from build123d import *

# Parameters (mm, degrees)
SKETCH1_R           = 12.25
BOSS_EXTRUDE1_DEPTH = 2.9
CUT_EXTRUDE1_REACH  = 364.631
SKETCH2_R           = 5
CUT_EXTRUDE2_REACH  = 364.631
SKETCH5_R           = 1.65
SKETCH6_R           = 9.75
SKETCH6_R_2         = 5
BOSS_EXTRUDE2_DEPTH = 3.72
SKETCH7_R           = 1.65
CUT_EXTRUDE3_DEPTH  = 3.72
SKETCH8_R           = 2.7
CUT_EXTRUDE4_DEPTH  = 2.5


with BuildPart() as part:
    # Sketch1 → Boss-Extrude1 (new body)
    with BuildSketch(Plane.XY):
        with Locations(Location((350.15, -0.367507575, 0), (0, 0, 180))):
            Circle(SKETCH1_R)
    extrude(amount=BOSS_EXTRUDE1_DEPTH)

    # Sketch2 → Cut-Extrude1 (cut, up to next)
    with BuildSketch(Plane.XY.offset(2.9), mode=Mode.PRIVATE) as cut_extrude1_sk1:
        with Locations((350.15, -0.367507575)):
            Circle(SKETCH2_R)
    cut_extrude1_tool1 = extrude(cut_extrude1_sk1.sketch, amount=-CUT_EXTRUDE1_REACH, mode=Mode.PRIVATE) & part.part
    add(cut_extrude1_tool1.solids().sort_by_distance((350.15, -0.367508, 2.9))[0], mode=Mode.SUBTRACT)

    # Sketch5 → Cut-Extrude2 (cut, up to next)
    with BuildSketch(Plane.XY.offset(2.9), mode=Mode.PRIVATE) as cut_extrude2_sk1:
        with Locations((343.05020627, -2.784722708)):
            Circle(SKETCH5_R)
    cut_extrude2_tool1 = extrude(cut_extrude2_sk1.sketch, amount=-CUT_EXTRUDE2_REACH, mode=Mode.PRIVATE) & part.part
    # Sketch5 → Cut-Extrude2 (cut, up to next)
    with BuildSketch(Plane.XY.offset(2.9), mode=Mode.PRIVATE) as cut_extrude2_sk2:
        with Locations((355.793266576, -5.30750174)):
            Circle(SKETCH5_R)
    cut_extrude2_tool2 = extrude(cut_extrude2_sk2.sketch, amount=-CUT_EXTRUDE2_REACH, mode=Mode.PRIVATE) & part.part
    # Sketch5 → Cut-Extrude2 (cut, up to next)
    with BuildSketch(Plane.XY.offset(2.9), mode=Mode.PRIVATE) as cut_extrude2_sk3:
        with Locations((351.606527153, 6.989701723)):
            Circle(SKETCH5_R)
    cut_extrude2_tool3 = extrude(cut_extrude2_sk3.sketch, amount=-CUT_EXTRUDE2_REACH, mode=Mode.PRIVATE) & part.part
    add(cut_extrude2_tool1.solids().sort_by_distance((343.050206, -2.784723, 2.9))[0], mode=Mode.SUBTRACT)
    add(cut_extrude2_tool2.solids().sort_by_distance((355.793267, -5.307502, 2.9))[0], mode=Mode.SUBTRACT)
    add(cut_extrude2_tool3.solids().sort_by_distance((351.606527, 6.989702, 2.9))[0], mode=Mode.SUBTRACT)

    # Sketch6 → Boss-Extrude2 (add)
    with BuildSketch(Plane(origin=(0, 0, 0), x_dir=(-1, 0, 0), z_dir=(0, 0, -1))):
        with Locations(Location((-350.15, -0.367507575, 0), (0, 0, 180))):
            Circle(SKETCH6_R)
        with Locations(Location((-350.15, -0.367507575, 0), (0, 0, 180))):
            Circle(SKETCH6_R_2, mode=Mode.SUBTRACT)
    extrude(amount=BOSS_EXTRUDE2_DEPTH)

    # Sketch7 → Cut-Extrude3 (cut)
    with BuildSketch(Plane.XY):
        with Locations((351.606527153, 6.989701723)):
            Circle(SKETCH7_R)
        with Locations((343.05020627, -2.784722708)):
            Circle(SKETCH7_R)
        with Locations((355.793266576, -5.30750174)):
            Circle(SKETCH7_R)
    extrude(amount=-CUT_EXTRUDE3_DEPTH, mode=Mode.SUBTRACT)

    # Sketch8 → Cut-Extrude4 (cut)
    with BuildSketch(Plane.XY.offset(2.9)):
        with Locations((351.606527153, 6.989701723)):
            Circle(SKETCH8_R)
        with Locations((355.793266576, -5.30750174)):
            Circle(SKETCH8_R)
        with Locations((343.05020627, -2.784722708)):
            Circle(SKETCH8_R)
    extrude(amount=-CUT_EXTRUDE4_DEPTH, mode=Mode.SUBTRACT)


solid = part.part
CAD build for the part. Positions are in the model's coordinates, mm. A direction names the side the tool comes from. Round coordinates to 2 decimals unless told otherwise and drop trailing zeros. Loops run counter-clockwise (first coordinate to the right, second up) from the corner with the lowest first, then second, coordinate; pieces in that order, holes last.
(1) Cut at D-D (x = 350.75). Give the cut face in (y, z), plus the area to 3 significant figures.
(2) Two-plate mould, pull along Y, no slides. Class faces 1 (the cylindrical face through (354.92, -1.87, -0.36)), 2 (the flat face through (351, 10, 0)), 3 (the cylindrical face through (340.41, -0.8, -1.83)), 4 (the cylindrical face through (341.4, -2.71, -1.63)): +Y half, -Y half, draft (parallel to the pull), parting line (faces both ways), or undercut.
(3) Which spindle directions (+Z, -Z, +X, -X, +Y, -Y) get a long thin tool onto all of the face, cutting with end or side? Do faces 5 (the flat face through (343, -5, 0.4)), 6 (the cylindrical face through (353.18, 7.49, -1.63)). Say none if no direction does.
(4) Cut at A-A (y = 0.5). Give the cut face in (x, z), plus the area to 3 significant figures.
(5) Wall check: line 1 along X through (y, z) = (-1.75, -1.5); line 2 along Y through (x, z) = (353.5, 2.25); line 3 along Y through (x, z) = (352.25, -3.5). Give the ranges that are in metal, low to high.
(6) Cut at B-B (x = 353.75). Give the cut face in (y, z), plus the area to 3 significant figures.
(7) Drop flat-ended pins along their axis: pin 1 (1 mm diameter, centred on y = 7.5, z = 0, fed in from +X); pin 2 (2 mm diameter, centred on x = 355.79, y = -5.31, fed in from +Z); pin 3 (1.5 mm diameter, centred on x = 341.5, y = 8.5, fed in from -Z); pin 4 (4.5 mm diameter, centred on x = 351.61, y = 6.99, fed in from +Z). Give the stop position or say it passes through.
Findings below:
1. outline: (-12.6, 0) - (-10.1, 0) - (-10.1, -3.72) - (-5.33, -3.72) - (-5.33, 2.9) - (-12.6, 2.9) - close; (4.6, -3.72) - (5.58, -3.72) - (5.58, 0.4) - (4.6, 0.4) - close; (8.4, -3.72) - (9.36, -3.72) - (9.36, 0) - (11.87, 0) - (11.87, 2.9) - (9.55, 2.9) - (9.55, 0.4) - (8.4, 0.4) - close
1. area: 53.6 mm2
2. face 1: undercut
2. face 2: draft
2. face 3: parting line
2. face 4: undercut
3. face 5: +Z
3. face 6: +Z, -Z
4. outline: (337.93, 0) - (340.44, 0) - (340.44, -3.72) - (345.23, -3.72) - (345.23, 2.9) - (337.93, 2.9) - close; (355.07, -3.72) - (359.86, -3.72) - (359.86, 0) - (362.37, 0) - (362.37, 2.9) - (355.07, 2.9) - close
4. area: 77.9 mm2
5. line 1: x = 340.5 to 341.76, 344.34 to 345.34, 354.96 to 359.8
5. line 2: y = -12.15 to -6.73, 3.34 to 5.06, 8.91 to 11.42
5. line 3: y = -9.89 to -4.91, 4.17 to 5.47, 8.51 to 9.15
6. outline: (-12.08, 0) - (-9.43, 0) - (-9.43, -3.72) - (-3.84, -3.72) - (-3.84, 0.4) - (-7.07, 0.4) - (-7.07, 2.9) - (-12.08, 2.9) - close; (3.1, -3.72) - (8.69, -3.72) - (8.69, 0) - (11.34, 0) - (11.34, 2.9) - (8.63, 2.9) - (8.63, 0.4) - (5.35, 0.4) - (5.35, 2.9) - (3.1, 2.9) - close
6. area: 73.1 mm2
7. pin 1: stops at x = 359.94
7. pin 2: passes through
7. pin 3: stops at z = 0
7. pin 4: stops at z = 0.4
